from build123d import *

# Parameters (mm, degrees)
F0_W     = 33.4264
F0_H     = 6.774552
F1_DEPTH = 1.27
F3_D     = 2.54
F4_R     = 1.116582
F5_DEPTH = 5.7658
F7_R     = 1.207406
F8_DEPTH = 5.08


with BuildPart() as f1:
    # F0 (on Top) → F1 (new body)
    with BuildSketch(Plane.XY):
        with Locations((-32.106044, -54.848913)):
            Rectangle(F0_W, F0_H)
    extrude(amount=F1_DEPTH)

    # F3 (through all)
    with Locations(Plane.XY.offset(1.27)):
        with Locations((-37.410062, -55.545177)):
            Hole(F3_D / 2)

    # F7 (on face) → F8 (join)
    with BuildSketch(Plane.XY.offset(1.27)):
        with Locations((-43.920558, -54.636113)):
            Circle(F7_R)
    extrude(amount=F8_DEPTH)


with BuildPart() as f5:
    # F4 (on face) → F5 (new body)
    with BuildSketch(Plane.XY.offset(1.27)):
        with Locations((-37.410062, -55.545177)):
            Circle(F4_R)
    extrude(amount=F5_DEPTH)


solid = f1.part
The model under review builds one solid part; all positions refer to its coordinate system, in mm. A direction names the side the tool comes from. Round coordinates to 2 decimals unless told otherwise and drop trailing zeros. Write each loop counter-clockwise with the first axis right and the second up, starting at its lowest first coordinate (ties: lowest second). Pieces come first, ordered by that corner, then holes. Notation, with made-up numbers: (37.5, -35.75) -> (82.5, -35.75) arc R20 ccw to (82.5, -27.75) -> close; hole circle Ø2 at (-11, 9.25). An arc over 180 degrees is marked (long way). Answer as a JSON object with one key per item and string values.
1. We need section D-D on x = -43.5. State the section outline as (y, z) points, and give its area (3 significant figures).
Results found:
{"outline": "(-58.24, 0) -> (-51.46, 0) -> (-51.46, 1.27) -> (-53.5, 1.27) -> (-53.5, 6.35) -> (-55.77, 6.35) -> (-55.77, 1.27) -> (-58.24, 1.27) -> close", "area": "20.1 mm^2"}
2. The part is to be moulded in two halves that separate along X. For faces 1 (the face through (-38, -56.67, 0.63)), 2 (the face through (-32, -55, 0)), 3 (the face through (-48.819, -55, 1)), 4 (the face through (-15.393, -55, 1)), say which applies: pulls with the +X half, pulls with the -X half, needs draft (parallel to the pull), parting line crosses it, or undercut.
Results found:
{"face 1": "undercut", "face 2": "needs draft", "face 3": "pulls with the -X half", "face 4": "pulls with the +X half"}
3. To check wall thickness, follow line 1 along Z through (x, y) = (-39, -55.5); line 2 along X through (y, z) = (-55.5, 1); line 3 along X through (y, z) = (-54.75, 5.5). State the ranges of each line that lie inside material, in increasing order.
Results found:
{"line 1": "z = 0 to 1.27", "line 2": "x = -48.82 to -38.68, -36.14 to -15.39", "line 3": "x = -45.12 to -42.72"}
4. We need section C-C on y = -53. State the section outline as (x, z) points, and give its area (3 significant figures).
Results found:
{"outline": "(-48.82, 0) -> (-15.39, 0) -> (-15.39, 1.27) -> (-48.82, 1.27) -> close", "area": "42.5 mm^2"}
5. We need section B-B on y = -56.25. State the section outline as (x, z) points, and give its area (3 significant figures).
Results found:
{"outline": "(-48.82, 0) -> (-38.47, 0) -> (-38.47, 1.27) -> (-48.82, 1.27) -> close; (-36.35, 0) -> (-15.39, 0) -> (-15.39, 1.27) -> (-36.35, 1.27) -> close", "area": "39.8 mm^2"}
6. Machinability: for faces 5 (the face through (-44.88, -55.37, 3.77)), 6 (the face through (-44, -55, 6.35)), which of the approach directions +Z, -Z, +X, -X, +Y, -Y give a long, thin tool a straight path to every point of the face, cutting with its end or side? Answer none if there is none.
Results found:
{"face 5": "+Z", "face 6": "+Z, +X, -X, +Y, -Y"}
7. Clearance check with flat-ended pins moving along their axes: pin 1 (1.5 mm diameter, centred on x = -38, y = -57, fed in from -Z); pin 2 (3 mm diameter, centred on y = -57, z = 3, fed in from +X). State where each tip first meets the part, or that it passes through.
Results found:
{"pin 1": "stops at z = 0", "pin 2": "stops at x = -43.08"}
8. We need section A-A on x = -37. State the section outline as (y, z) points.
Results found:
{"outline": "(-58.24, 0) -> (-56.75, 0) -> (-56.75, 1.27) -> (-58.24, 1.27) -> close; (-54.34, 0) -> (-51.46, 0) -> (-51.46, 1.27) -> (-54.34, 1.27) -> close"}
